Read the model definition and answer for the solid it produces. Units are mm, in the model's axes. A direction names the side the tool comes from. Coordinates: 2 decimals unless noted, no trailing zeros. One line per item, written item: value. Start each with the question number.
1. Flat-ended cylindrical pins translate along their axes: pin 1 (3.5 mm diameter, centred on x = -23.5, y = -25, fed in from -Z); pin 2 (1.9 mm diameter, centred on x = -18, z = 5, fed in from -Y). Find the tip coordinate at first contact, or state that the pin passes through.
2. The part is cut by section A-A (z = 6.35). State how many separate pieces and enclosed holes the cut face has, then the cut area to 3 significant figures.
3. Consider probe 1 along Y at (x, z) = (0, 10.5); probe 2 along Z at (x, y) = (26, 23). Determine where each line is inside the solid, lowest interval first.
4. Determine the mould class of faces 4 (the face through (-29.94, -29.84, 6.44)), 5 (the face through (20.53, -25.49, 7.3)), 6 (the face through (23, -24, 12.7)) for opening direction X: +X half, -X half, draft (parallel to the pull), parting line (faces both ways), or undercut.
5. For faces 1 (the face through (-6.883, 30.995, 13.866)), 2 (the face through (26.615, -21.895, 1.972)), 3 (the face through (-14.57, 25.49, 7.57)), determine the directions among +Z, -Z, +X, -X, +Y, -Y from which every point of the face is accessible in a straight line to the end or side of a thin tool.
Autodesk Inventor part; units mm, degrees
ref_plane "YZ Plane" through (0, 0, 0) normal (1, 0, 0) x (0, 1, 0)
ref_plane "XZ Plane" through (0, 0, 0) normal (0, 1, 0) x (-1, 0, 0)
ref_plane "XY Plane" through (0, 0, 0) normal (0, 0, 1) x (1, 0, 0)
sketch "Sketch1" plane through (0, 0, 0) normal (0, 0, 1) x (1, 0, 0)
  circle A0 centre (0, 0) radius 14
  line L0 (-31.75, 31.75) -> (31.75, 31.75)
  line L1 (31.75, 31.75) -> (31.75, -31.75)
  line L2 (31.75, -31.75) -> (-31.75, -31.75)
  line L3 (-31.75, -31.75) -> (-31.75, 31.75)
  circle A1 centre (0, 27.0002) radius 2.3495
  line L4 (-31.75, 0) -> (31.75, 0) construction
  line L5 (0, 31.75) -> (0, -31.75) construction
  circle A2 centre (-27.0002, 0) radius 2.3495
  circle A3 centre (27.0002, 0) radius 2.3495
  circle A4 centre (0, -27.0002) radius 2.3495
  circle A5 centre (-25.0002, 25.0002) radius 2
  line L6 (-27.0002, -27.0002) -> (27.0002, -27.0002) construction
  line L7 (27.0002, -27.0002) -> (27.0002, 27.0002) construction
  line L8 (27.0002, 27.0002) -> (-27.0002, 27.0002) construction
  line L9 (-27.0002, 27.0002) -> (-27.0002, -27.0002) construction
  circle A6 centre (-25.0002, 25.0002) radius 3.5
  circle A7 centre (25.0002, 25.0002) radius 2
  circle A8 centre (25.0002, 25.0002) radius 3.5
  circle A9 centre (-25.0002, -25.0002) radius 2
  circle A10 centre (-25.0002, -25.0002) radius 3.5
  circle A11 centre (25.0002, -25.0002) radius 2
  circle A12 centre (25.0002, -25.0002) radius 3.5
  dimension "d2" = 28
  dimension "d7" = 63.5
  dimension "d8" = 63.5
  dimension "d9" = 27.0002
  dimension "d10" = 4.699
  dimension "d11" = 27.0002
  dimension "d12" = 27.0002
  dimension "d13" = 27.0002
  dimension "d14" = 54.0004
  dimension "d17" = 4
  dimension "d18" = 7
extrude "Extrusion1" add sketch "Sketch1" along normal blind 12.7 contours L0 L1 L2 L3 | A6 | A8 | A10 | A12
extrude "Extrusion2" cut sketch "Sketch1" along normal blind 4 contours A6 | A8 | A10 | A12
fillet "Fillet1" radius 6.35 4 edges at (31.75, 31.75, 6.35) (-31.75, 31.75, 6.35) (31.75, -31.75, 6.35) (-31.75, -31.75, 6.35)
sketch "Sketch2" plane through (0, 0, 12.7) normal (0, 0, 1) x (1, 0, 0)
  circle A0 centre (0, 0) radius 14
  circle A1 centre (0, -27.0002) radius 2.3495
  circle A2 centre (27.0002, 0) radius 2.3495
  circle A3 centre (-27.0002, 0) radius 2.3495
  circle A4 centre (0, 27.0002) radius 2.3495
  circle A5 centre (0, 0) radius 31.75
  dimension "d22" = 63.5
extrude "Extrusion3" add sketch "Sketch2" along normal blind 3
sketch "Sketch3" plane through (0, 0, 15.7) normal (0, 0, 1) x (1, 0, 0)
  circle A0 centre (0, 0) radius 14
  circle A1 centre (27.0002, 0) radius 2.3495
  circle A2 centre (0, 0) radius 31.75
  circle A3 centre (0, 0) radius 24.6507
extrude "Extrusion4" add sketch "Sketch3" along normal blind 2 contours A3
thread "Thread1"
thread "Thread2"
thread "Thread3"
thread "Thread4"
chamfer "Chamfer1" distance 0.635 angle 45 1 edges at (-31.75, 0, 15.7)
sketch "Sketch4" plane through (-25.4, 31.75, 0) normal (0, 1, 0) x (1, 0, 0)
  line L0 (50.8, -12.7) -> (25.4, -12.7)
  line L1 (25.4, 0) -> (25.4, -12.7) construction
  line L2 (7.8994, -6.35) -> (42.9006, -6.35) construction
  circle A0 centre (7.8994, -6.35) radius 3.175
  circle A1 centre (42.9006, -6.35) radius 3.175
  point P0 (25.4, -6.35)
  dimension "d38" = 35.0012
  dimension "d40" = 6.35
extrude "Extrusion5" cut sketch "Sketch4" against normal blind 12.7
sketch "Sketch5" plane through (-25.4, -31.75, 0) normal (0, -1, 0) x (1, 0, 0)
  line L0 (0, 12.7) -> (25.4, 12.7)
  line L1 (25.4, 0) -> (25.4, 12.7) construction
  line L2 (7.8994, 6.35) -> (42.9006, 6.35) construction
  circle A0 centre (7.8994, 6.35) radius 3.175
  circle A1 centre (42.9006, 6.35) radius 3.175
  point P0 (25.4, 6.35)
  dimension "d43" = 35.0012
  dimension "d45" = 6.35
extrude "Extrusion6" cut sketch "Sketch5" against normal blind 12.7
thread "Thread5"
thread "Thread6"
thread "Thread7"
thread "Thread8"
properties part number "P80 Front Block" material "Steel"
Answer block:
1. pin 1: stops at z = 4
1. pin 2: stops at y = -19.05
2. separate pieces: 1
2. enclosed holes: 9
2. area: 2,940 mm2
3. probe 1: y = -31.75 to -29.35, -24.65 to -14, 14 to 24.65, 29.35 to 31.75
3. probe 2: z = 4 to 12.7
4. face 4: -X half
4. face 5: undercut
4. face 6: draft
5. face 1: +Z
5. face 2: -Z
5. face 3: +Y
